from build123d import *

# Parameters (mm, degrees)
SKETCH_1_W          = 444
SKETCH_1_H          = 1106
EXTRUDE_305_DEPTH   = 64
CUT_EXTRUDE_1_DEPTH = 42


with BuildPart() as part:
    # Эскиз1 → Extrude 305 (new body)
    with BuildSketch(Plane(origin=(0, 0, 0), x_dir=(1, 0, 0), z_dir=(0, 1, 0))):
        with Locations((222, 553)):
            Rectangle(SKETCH_1_W, SKETCH_1_H)
    extrude(amount=-EXTRUDE_305_DEPTH)

    # Эскиз2 → Вырез-Вытянуть1 (cut)
    with BuildSketch(Plane(origin=(0, 0, 0), x_dir=(1, 0, 0), z_dir=(0, 1, 0))):
        Polygon((222, 1015.363466897), (77, 1015.363466897), (77, 905.636533103), (222, 905.636533103), (367, 905.636533103), (367, 1015.363466897), align=None)
        Polygon((222, 852.363466897), (92, 852.363466897), (92, 742.636533103), (222, 742.636533103), (352, 742.636533103), (352, 852.363466897), align=None)
        Polygon((222, 689.363466897), (92, 689.363466897), (92, 579.636533103), (222, 579.636533103), (352, 579.636533103), (352, 689.363466897), align=None)
        Polygon((222, 526.363466897), (92, 526.363466897), (92, 416.636533103), (222, 416.636533103), (352, 416.636533103), (352, 526.363466897), align=None)
        Polygon((222, 363.363466897), (92, 363.363466897), (92, 253.636533103), (222, 253.636533103), (352, 253.636533103), (352, 363.363466897), align=None)
        Polygon((222, 200.363466897), (127, 200.363466897), (127, 90.636533103), (222, 90.636533103), (317, 90.636533103), (317, 200.363466897), align=None)
    extrude(amount=-CUT_EXTRUDE_1_DEPTH, mode=Mode.SUBTRACT)


solid = part.part
Source: CAD feature listing. Evaluate the final solid. Frame: model axes, mm. A direction names the side the tool comes from. Round coordinates to 2 decimals unless told otherwise and drop trailing zeros. Loops run counter-clockwise (first coordinate to the right, second up) from the corner with the lowest first, then second, coordinate; pieces in that order, holes last. Notation, with made-up numbers: M -21.75,17 L 26.25,17 A19 cw 26.25,28 Z; hole C -29.5,-4.5 d9. An arc over 180 degrees is marked long. Return JSON: item names as keys, results as strings. Group by question number.
1. Section query A-A on y = -14. Output: boundary loops of the cut face in (x, z), and give its area (3 significant figures).
2. Section query C-C on x = 186. Output: boundary loops of the cut face in (y, z), and give its area (3 significant figures).
3. Material intervals for line 1 along X through (y, z) = (-21.5, -654); line 2 along X through (y, z) = (-31, -107.5); line 3 along Y through (x, z) = (303, -616), sorted ascending. Write a range as from..to.
4. Section query D-D on z = -630.5. Output: boundary loops of the cut face in (x, y), and give its area (3 significant figures).
5. Reachability of faces 1 (the face through (317, -21, -145)), 2 (the face through (0, -32, -545)) from +Z, -Z, +X, -X, +Y, -Y: full face, straight path, thin tool, end or side. Return the list, or none.
6. Section query B-B on z = -969. Output: boundary loops of the cut face in (x, y).
7. Pin query (flat end, axial travel): pin 1 (3 mm diameter, centred on x = 224, y = -10, fed in from +Z). Return the tip coordinate at first contact, or that it passes through.
Checks:
{
 "1": {"outline": "M 0,-1106 L 444,-1106 L 444,0 L 0,0 Z; hole M 77,-1015.36 L 367,-1015.36 L 367,-905.64 L 77,-905.64 Z; hole M 92,-852.36 L 352,-852.36 L 352,-742.64 L 92,-742.64 Z; hole M 92,-689.36 L 352,-689.36 L 352,-579.64 L 92,-579.64 Z; hole M 92,-526.36 L 352,-526.36 L 352,-416.64 L 92,-416.64 Z; hole M 92,-363.36 L 352,-363.36 L 352,-253.64 L 92,-253.64 Z; hole M 127,-200.36 L 317,-200.36 L 317,-90.64 L 127,-90.64 Z", "area": "324,000 mm²"},
 "2": {"outline": "M -64,-1106 L 0,-1106 L 0,-1015.36 L -42,-1015.36 L -42,-905.64 L 0,-905.64 L 0,-852.36 L -42,-852.36 L -42,-742.64 L 0,-742.64 L 0,-689.36 L -42,-689.36 L -42,-579.64 L 0,-579.64 L 0,-526.36 L -42,-526.36 L -42,-416.64 L 0,-416.64 L 0,-363.36 L -42,-363.36 L -42,-253.64 L 0,-253.64 L 0,-200.36 L -42,-200.36 L -42,-90.64 L 0,-90.64 L 0,0 L -64,0 Z", "area": "43,100 mm²"},
 "3": {"line 1": "x = 0..92, 352..444", "line 2": "x = 0..127, 317..444", "line 3": "y = -64..-42"},
 "4": {"outline": "M 0,-64 L 444,-64 L 444,0 L 352,0 L 352,-42 L 92,-42 L 92,0 L 0,0 Z", "area": "17,500 mm²"},
 "5": {"face 1": "+Y", "face 2": "+Z, -Z, -X, +Y, -Y"},
 "6": {"outline": "M 0,-64 L 444,-64 L 444,0 L 367,0 L 367,-42 L 77,-42 L 77,0 L 0,0 Z"},
 "7": {"pin 1": "stops at z = 0"}
}
